from build123d import *

# Parameters (mm, degrees)
SKETCH1_W              = 69.85
SKETCH1_H              = 50.8
BASE_DEPTH             = 3.81
PHONE_SUPPORT_DEPTH    = 69.85
FRONT_FACE_CUT_DEPTH   = 88.719987912
SKETCH4_W              = 59.563
SKETCH4_H              = 8.7122
PHONE_SLOT_DEPTH       = 10.16
HOME_BUTTON_HOLE_REACH = 87.363
FILLET1_R              = 3.81
FILLET2_R              = 3.048


with BuildPart() as part:
    # Sketch1 → Base (new body)
    with BuildSketch(Plane(origin=(0, 0, 0), x_dir=(1, 0, 0), z_dir=(0, 1, 0))):
        with Locations((34.925, 25.4)):
            Rectangle(SKETCH1_W, SKETCH1_H)
    extrude(amount=BASE_DEPTH)

    # Sketch2 → Phone support (add, through all)
    with BuildSketch(Plane(origin=(69.85, 0, 0), x_dir=(0, 0, -1), z_dir=(1, 0, 0))):
        Polygon((33.922616542, 3.81), (49.779113577, 3.81), (46.691247659, 15.334072492), (31.896934518, 11.369948234), align=None)
    extrude(amount=-PHONE_SUPPORT_DEPTH)

    # Sketch3 → Front face cut (cut, through all)
    with BuildSketch(Plane(origin=(69.85, 0, 0), x_dir=(0, 0, -1), z_dir=(1, 0, 0))):
        Polygon((50.8, 0), (49.779113577, 3.81), (50.8, 3.81), align=None)
    extrude(amount=-FRONT_FACE_CUT_DEPTH, mode=Mode.SUBTRACT)

    # Sketch4 → Phone slot (cut)
    with BuildSketch(Plane(origin=(0, 2.634072492, 0.705797597), x_dir=(1, 0, 0), z_dir=(0, 0.96592582628907, 0.2588190451025147))):
        with Locations((34.925, 41.410931975)):
            Rectangle(SKETCH4_W, SKETCH4_H)
    extrude(amount=-PHONE_SLOT_DEPTH, mode=Mode.SUBTRACT)

    # Sketch5 → Home button hole (cut, up to next)
    with BuildSketch(Plane(origin=(0, 12.7, -47.397045256), x_dir=(-1, 0, 0), z_dir=(0, 0.2588190451025147, -0.96592582628907)), mode=Mode.PRIVATE) as home_button_hole_sk1:
        with BuildLine():
            ThreePointArc((-43.17999875, 1.406192509), (-40.762165229, -4.43097397), (-34.92499875, -6.848807491))
            Line((-34.92499875, -6.848807491), (-34.92499875, 1.406192509))
            Line((-34.92499875, 1.406192509), (-43.17999875, 1.406192509))
        make_face()
    home_button_hole_tool1 = extrude(home_button_hole_sk1.sketch, amount=-HOME_BUTTON_HOLE_REACH, mode=Mode.PRIVATE) & part.part
    # Sketch5 → Home button hole (cut, up to next)
    with BuildSketch(Plane(origin=(0, 12.7, -47.397045256), x_dir=(-1, 0, 0), z_dir=(0, 0.2588190451025147, -0.96592582628907)), mode=Mode.PRIVATE) as home_button_hole_sk2:
        with BuildLine():
            Line((-34.92499875, 1.406192509), (-34.92499875, -6.848807491))
            ThreePointArc((-34.92499875, -6.848807491), (-29.087832271, -4.43097397), (-26.66999875, 1.406192509))
            Line((-26.66999875, 1.406192509), (-34.92499875, 1.406192509))
        make_face()
    home_button_hole_tool2 = extrude(home_button_hole_sk2.sketch, amount=-HOME_BUTTON_HOLE_REACH, mode=Mode.PRIVATE) & part.part
    # Sketch5 → Home button hole (cut, up to next)
    with BuildSketch(Plane(origin=(0, 12.7, -47.397045256), x_dir=(-1, 0, 0), z_dir=(0, 0.2588190451025147, -0.96592582628907)), mode=Mode.PRIVATE) as home_button_hole_sk3:
        with BuildLine():
            ThreePointArc((-43.17999875, 1.406192509), (-40.762165229, -4.43097397), (-34.92499875, -6.848807491))
            Line((-34.92499875, -6.848807491), (-34.92499875, 1.406192509))
            Line((-34.92499875, 1.406192509), (-43.17999875, 1.406192509))
        make_face()
    home_button_hole_tool3 = extrude(home_button_hole_sk3.sketch, amount=-HOME_BUTTON_HOLE_REACH, mode=Mode.PRIVATE) & part.part
    # Sketch5 → Home button hole (cut, up to next)
    with BuildSketch(Plane(origin=(0, 12.7, -47.397045256), x_dir=(-1, 0, 0), z_dir=(0, 0.2588190451025147, -0.96592582628907)), mode=Mode.PRIVATE) as home_button_hole_sk4:
        with BuildLine():
            Line((-34.92499875, 1.406192509), (-34.92499875, -6.848807491))
            ThreePointArc((-34.92499875, -6.848807491), (-29.087832271, -4.43097397), (-26.66999875, 1.406192509))
            Line((-26.66999875, 1.406192509), (-34.92499875, 1.406192509))
        make_face()
    home_button_hole_tool4 = extrude(home_button_hole_sk4.sketch, amount=-HOME_BUTTON_HOLE_REACH, mode=Mode.PRIVATE) & part.part
    # Sketch5 → Home button hole (cut, up to next)
    with BuildSketch(Plane(origin=(0, 12.7, -47.397045256), x_dir=(-1, 0, 0), z_dir=(0, 0.2588190451025147, -0.96592582628907)), mode=Mode.PRIVATE) as home_button_hole_sk5:
        with BuildLine():
            Line((-43.17999875, 1.406192509), (-34.92499875, 1.406192509))
            Line((-34.92499875, 1.406192509), (-34.92499875, 2.726992509))
            Line((-34.92499875, 2.726992509), (-43.073649703, 2.726992509))
            ThreePointArc((-43.073649703, 2.726992509), (-43.153368534, 2.068729821), (-43.17999875, 1.406192509))
        make_face()
    home_button_hole_tool5 = extrude(home_button_hole_sk5.sketch, amount=-HOME_BUTTON_HOLE_REACH, mode=Mode.PRIVATE) & part.part
    # Sketch5 → Home button hole (cut, up to next)
    with BuildSketch(Plane(origin=(0, 12.7, -47.397045256), x_dir=(-1, 0, 0), z_dir=(0, 0.2588190451025147, -0.96592582628907)), mode=Mode.PRIVATE) as home_button_hole_sk6:
        with BuildLine():
            Line((-34.92499875, 2.726992509), (-34.92499875, 1.406192509))
            Line((-34.92499875, 1.406192509), (-26.66999875, 1.406192509))
            ThreePointArc((-26.66999875, 1.406192509), (-26.696628966, 2.068729821), (-26.776347797, 2.726992509))
            Line((-26.776347797, 2.726992509), (-34.92499875, 2.726992509))
        make_face()
    home_button_hole_tool6 = extrude(home_button_hole_sk6.sketch, amount=-HOME_BUTTON_HOLE_REACH, mode=Mode.PRIVATE) & part.part
    # Sketch5 → Home button hole (cut, up to next)
    with BuildSketch(Plane(origin=(0, 12.7, -47.397045256), x_dir=(-1, 0, 0), z_dir=(0, 0.2588190451025147, -0.96592582628907)), mode=Mode.PRIVATE) as home_button_hole_sk7:
        with BuildLine():
            Line((-43.17999875, 1.406192509), (-34.92499875, 1.406192509))
            Line((-34.92499875, 1.406192509), (-34.92499875, 2.726992509))
            Line((-34.92499875, 2.726992509), (-43.073649703, 2.726992509))
            ThreePointArc((-43.073649703, 2.726992509), (-43.153368534, 2.068729821), (-43.17999875, 1.406192509))
        make_face()
    home_button_hole_tool7 = extrude(home_button_hole_sk7.sketch, amount=-HOME_BUTTON_HOLE_REACH, mode=Mode.PRIVATE) & part.part
    # Sketch5 → Home button hole (cut, up to next)
    with BuildSketch(Plane(origin=(0, 12.7, -47.397045256), x_dir=(-1, 0, 0), z_dir=(0, 0.2588190451025147, -0.96592582628907)), mode=Mode.PRIVATE) as home_button_hole_sk8:
        with BuildLine():
            Line((-34.92499875, 2.726992509), (-34.92499875, 1.406192509))
            Line((-34.92499875, 1.406192509), (-26.66999875, 1.406192509))
            ThreePointArc((-26.66999875, 1.406192509), (-26.696628966, 2.068729821), (-26.776347797, 2.726992509))
            Line((-26.776347797, 2.726992509), (-34.92499875, 2.726992509))
        make_face()
    home_button_hole_tool8 = extrude(home_button_hole_sk8.sketch, amount=-HOME_BUTTON_HOLE_REACH, mode=Mode.PRIVATE) & part.part
    # Sketch5 → Home button hole (cut, up to next)
    with BuildSketch(Plane(origin=(0, 12.7, -47.397045256), x_dir=(-1, 0, 0), z_dir=(0, 0.2588190451025147, -0.96592582628907)), mode=Mode.PRIVATE) as home_button_hole_sk9:
        with BuildLine():
            Line((-43.17999875, 2.726992509), (-43.17999875, 1.406192509))
            ThreePointArc((-43.17999875, 1.406192509), (-43.153368534, 2.068729821), (-43.073649703, 2.726992509))
            Line((-43.073649703, 2.726992509), (-43.17999875, 2.726992509))
        make_face()
    home_button_hole_tool9 = extrude(home_button_hole_sk9.sketch, amount=-HOME_BUTTON_HOLE_REACH, mode=Mode.PRIVATE) & part.part
    # Sketch5 → Home button hole (cut, up to next)
    with BuildSketch(Plane(origin=(0, 12.7, -47.397045256), x_dir=(-1, 0, 0), z_dir=(0, 0.2588190451025147, -0.96592582628907)), mode=Mode.PRIVATE) as home_button_hole_sk10:
        with BuildLine():
            ThreePointArc((-26.776347797, 2.726992509), (-26.696628966, 2.068729821), (-26.66999875, 1.406192509))
            Line((-26.66999875, 1.406192509), (-26.66999875, 2.726992509))
            Line((-26.66999875, 2.726992509), (-26.776347797, 2.726992509))
        make_face()
    home_button_hole_tool10 = extrude(home_button_hole_sk10.sketch, amount=-HOME_BUTTON_HOLE_REACH, mode=Mode.PRIVATE) & part.part
    add(home_button_hole_tool1.solids().sort_by_distance((38.42853, 10.674127, -47.939876))[0], mode=Mode.SUBTRACT)
    add(home_button_hole_tool2.solids().sort_by_distance((31.421468, 10.674127, -47.939876))[0], mode=Mode.SUBTRACT)
    add(home_button_hole_tool3.solids().sort_by_distance((38.42853, 10.674127, -47.939876))[0], mode=Mode.SUBTRACT)
    add(home_button_hole_tool4.solids().sort_by_distance((31.421468, 10.674127, -47.939876))[0], mode=Mode.SUBTRACT)
    add(home_button_hole_tool5.solids().sort_by_distance((39.034881, 14.694801, -46.86254))[0], mode=Mode.SUBTRACT)
    add(home_button_hole_tool6.solids().sort_by_distance((30.815117, 14.694801, -46.86254))[0], mode=Mode.SUBTRACT)
    add(home_button_hole_tool7.solids().sort_by_distance((39.034881, 14.694801, -46.86254))[0], mode=Mode.SUBTRACT)
    add(home_button_hole_tool8.solids().sort_by_distance((30.815117, 14.694801, -46.86254))[0], mode=Mode.SUBTRACT)
    add(home_button_hole_tool9.solids().sort_by_distance((43.14813, 15.015536, -46.776599))[0], mode=Mode.SUBTRACT)
    add(home_button_hole_tool10.solids().sort_by_distance((26.701868, 15.015536, -46.776599))[0], mode=Mode.SUBTRACT)

    # Fillet1
    fillet1_edges = [part.edges().sort_by_distance(p)[0] for p in [
        (34.925, 3.81, -33.922616542),
    ]]
    fillet(fillet1_edges, radius=FILLET1_R)

    # Fillet2
    fillet2_edges = [part.edges().sort_by_distance(p)[0] for p in [
        (34.925, 3.81, 0),
    ]]
    fillet(fillet2_edges, radius=FILLET2_R)


solid = part.part
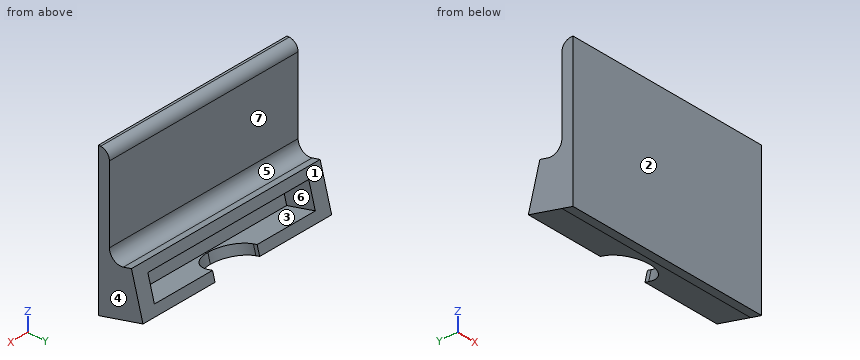
For this review, take the finished solid that the model builds, in its own axes (mm). Face numbers are marked on the shaded views. A direction names the side the tool comes from. Coordinates: 2 decimals unless noted, no trailing zeros. Order: outer loops, then holes, each group sorted by start corner. A loop starts at its lowest first (then second) coordinate and runs counter-clockwise, first axis right, second up. Notation, with made-up numbers: (32, 48.5) -> (91, 48.5) arc R19 ccw to (91, 58.5) -> close; hole circle Ø7 at (68.25, 62.25). An arc over 180 degrees is marked (long way). Return JSON: item names as keys, results as strings.
1. For pin 1 Ø1 at (x, z) = (33.5, -19.5) entering from +Y; pin 2 Ø4 at (x, y) = (12, 3) entering from +Z; pin 3 Ø1.5 at (x, z) = (39, -40.5) entering from +Y; pin 4 Ø5 at (y, z) = (7, -22) entering from +X, all flat-tipped, find the tip position at first contact; note any pin that passes through.
Answer block:
{"pin 1": "y = 3.81", "pin 2": "z = -0.01", "pin 3": "y = 3.36", "pin 4": "through"}
2. We need section B-B on z = -26. Write out the cut boundary in (x, y), and give its area (3 significant figures).
Answer block:
{"outline": "(0, 0) -> (69.85, 0) -> (69.85, 3.81) -> (0, 3.81) -> close", "area": "266 mm²"}
3. For line 1 (X direction, y = 4.5, z = -41); line 2 (Z direction, x = 51.5, y = 9.5); line 3 (Z direction, x = 17.5, y = 10), list the stretches that pass through material, from the lowest coordinate up. Write a range as from..to.
Answer block:
{"line 1": "0..5.14, 64.71..69.85", "line 2": "-48.25..-44.84, -35.82..-32.4", "line 3": "-48.12..-44.7, -35.68..-32.26"}
4. We need section A-A on x = 49. Write out the cut boundary in (y, z).
Answer block:
{"outline": "(0, -50.8) -> (15.33, -46.69) -> (14.48, -43.5) -> (4.67, -46.13) -> (2.41, -37.72) -> (12.22, -35.09) -> (11.37, -31.9) -> (8.61, -32.64) arc R3.81 cw to (3.81, -28.96) -> (3.81, -3.05) arc R3.05 ccw to (0.76, 0) -> (0, 0) -> close"}
5. We need section D-D on z = -40.5. Write out the cut boundary in (x, y), and give its area (3 significant figures).
Answer block:
{"outline": "(0, 0) -> (69.85, 0) -> (69.85, 13.68) -> (64.71, 13.68) -> (64.71, 3.16) -> (5.14, 3.16) -> (5.14, 13.68) -> (0, 13.68) -> close", "area": "329 mm²"}
6. The part is to be moulded in two halves that separate along Y. For the marked faces 1, 2, 3 and 4, say which applies: +Y half, -Y half, draft (parallel to the pull), parting line (faces both ways), or undercut.
Answer block:
{"face 1": "+Y half", "face 2": "-Y half", "face 3": "undercut", "face 4": "draft"}
7. Machinability: for the marked faces 5, 6 and 7, which of the approach directions +Z, -Z, +X, -X, +Y, -Y give a long, thin tool a straight path to every point of the face, cutting with its end or side? Answer none if there is none.
Answer block:
{"face 5": "+Z, +X, -X", "face 6": "none", "face 7": "+Z, +X, -X, +Y"}
8. We need section C-C on x = 32. Write out the cut boundary in (y, z).
Answer block:
{"outline": "(0, -50.8) -> (6.6, -49.03) -> (5.75, -45.84) -> (4.67, -46.13) -> (2.41, -37.72) -> (12.22, -35.09) -> (11.37, -31.9) -> (8.61, -32.64) arc R3.81 cw to (3.81, -28.96) -> (3.81, -3.05) arc R3.05 ccw to (0.76, 0) -> (0, 0) -> close"}
